Geometry check sheet. Reference: the model listing, model coordinates, mm. Face numbers are marked on the shaded views. A direction names the side the tool comes from. Give positions to 0.01 mm unless a question says otherwise; leave off trailing zeros. Write each loop counter-clockwise with the first axis right and the second up, starting at its lowest first coordinate (ties: lowest second). Pieces come first, ordered by that corner, then holes. Notation, with made-up numbers: M 69,57.25 L 127,57.25 A17 cw 127,69.25 Z; hole C -22,-1.5 d11. An arc over 180 degrees is marked long. Write each question's results on one line, items separated by ' | '.
```python
from build123d import *

# Parameters (mm, degrees)
RESSALTO_EXTRUS_O1_DEPTH = 28.35
ESBO_O3_W                = 36.7
ESBO_O3_H                = 41.8
RESSALTO_EXTRUS_O2_DEPTH = 14.75
ESBO_O5_W                = 30.5
ESBO_O5_H                = 20.5
CORTE_EXTRUS_O2_DEPTH    = 13.2
CORTE_EXTRUS_O3_DEPTH    = 69.850889609
ESBO_O7_W                = 5
ESBO_O7_H                = 16.7
CORTE_EXTRUS_O4_DEPTH    = 6.5
FILETE1_R                = 2.5
ESBO_O8_W                = 8.5
ESBO_O8_H                = 3.5
CORTE_EXTRUS_O5_DEPTH    = 14
ESBO_O9_W                = 3.2
ESBO_O9_H                = 3.2
RESSALTO_EXTRUS_O3_DEPTH = 2
ESBO_O10_R               = 10.65
RESSALTO_EXTRUS_O4_DEPTH = 17
ESBO_O11_R               = 4.25
CORTE_EXTRUS_O6_DEPTH    = 25


with BuildPart() as part:
    # Esboço1 → Ressalto-extrusão1 (new body)
    with BuildSketch(Plane.XY):
        with BuildLine():
            Line((14.1, -8.525), (14.1, 22.625))
            Line((14.1, 22.625), (-14.1, 22.625))
            Line((-14.1, 22.625), (-14.1, -8.525))
            ThreePointArc((-14.1, -8.525), (0, -22.625), (14.1, -8.525))
        make_face()
    extrude(amount=RESSALTO_EXTRUS_O1_DEPTH)

    # Esboço3 → Ressalto-extrusão2 (add)
    with BuildSketch(Plane(origin=(0, 22.625, 0), x_dir=(1, 0, 0), z_dir=(0, 1, 0))):
        with Locations((0, -7.45)):
            Rectangle(ESBO_O3_W, ESBO_O3_H)
    extrude(amount=RESSALTO_EXTRUS_O2_DEPTH)

    # Esboço5 → Corte-extrusão2 (cut)
    with BuildSketch(Plane(origin=(0, 37.375, 0), x_dir=(1, 0, 0), z_dir=(0, 1, 0))):
        with Locations((0, -13.5)):
            Rectangle(ESBO_O5_W, ESBO_O5_H)
    extrude(amount=-CORTE_EXTRUS_O2_DEPTH, mode=Mode.SUBTRACT)

    # Esboço6 → Corte-extrusão3 (cut, through all)
    with BuildSketch(Plane(origin=(0, 37.375, 0), x_dir=(1, 0, 0), z_dir=(0, 1, 0))):
        with BuildLine():
            Line((-2, 13.45), (-2, 6.30835312))
            ThreePointArc((-2, 6.30835312), (0, 4.30835312), (2, 6.30835312))
            Line((2, 6.30835312), (2, 13.45))
            Line((2, 13.45), (-2, 13.45))
        make_face()
    extrude(amount=-CORTE_EXTRUS_O3_DEPTH, mode=Mode.SUBTRACT)

    # Esboço7 → Corte-extrusão4 (cut)
    with BuildSketch(Plane(origin=(0, 37.375, 0), x_dir=(1, 0, 0), z_dir=(0, 1, 0))):
        with Locations((-9.55, 5.1)):
            Rectangle(ESBO_O7_W, ESBO_O7_H)
        with Locations((9.55, 5.1)):
            Rectangle(ESBO_O7_W, ESBO_O7_H)
    extrude(amount=-CORTE_EXTRUS_O4_DEPTH, mode=Mode.SUBTRACT)

    # Filete1
    filete1_edges = [part.edges().sort_by_distance(p)[0] for p in [
        (-12.05, 30.875, -5.1),
        (-7.05, 30.875, -5.1),
        (7.05, 30.875, -5.1),
        (12.05, 30.875, -5.1),
    ]]
    fillet(filete1_edges, radius=FILETE1_R - 0.0001)  # a hair under: the kernel refuses the full size

    # Esboço8 → Corte-extrusão5 (cut)
    with BuildSketch(Plane(origin=(0, 0, -13.45), x_dir=(-1, 0, 0), z_dir=(0, 0, -1))):
        with Locations((0.04245602, 30)):
            Rectangle(ESBO_O8_W, ESBO_O8_H)
    extrude(amount=-CORTE_EXTRUS_O5_DEPTH, mode=Mode.SUBTRACT)

    # Esboço9 → Ressalto-extrusão3 (add)
    with BuildSketch(Plane(origin=(0, 37.375, 0), x_dir=(1, 0, 0), z_dir=(0, 1, 0))):
        with Locations((-13.65, -1.65)):
            Rectangle(ESBO_O9_W, ESBO_O9_H)
        with Locations((13.65, -1.65)):
            Rectangle(ESBO_O9_W, ESBO_O9_H)
    extrude(amount=RESSALTO_EXTRUS_O3_DEPTH)

    # Esboço10 → Ressalto-extrusão4 (add)
    with BuildSketch(Plane(origin=(0, 0, 0), x_dir=(-1, 0, 0), z_dir=(0, 0, -1))):
        with Locations(Location((0, -9.125, 0), (0, 0, 180))):
            Circle(ESBO_O10_R)
    extrude(amount=RESSALTO_EXTRUS_O4_DEPTH)

    # Esboço11 → Corte-extrusão6 (cut)
    with BuildSketch(Plane(origin=(0, 0, -17), x_dir=(-1, 0, 0), z_dir=(0, 0, -1))):
        with Locations((0, -9.125)):
            Circle(ESBO_O11_R)
    extrude(amount=-CORTE_EXTRUS_O6_DEPTH, mode=Mode.SUBTRACT)


solid = part.part
```
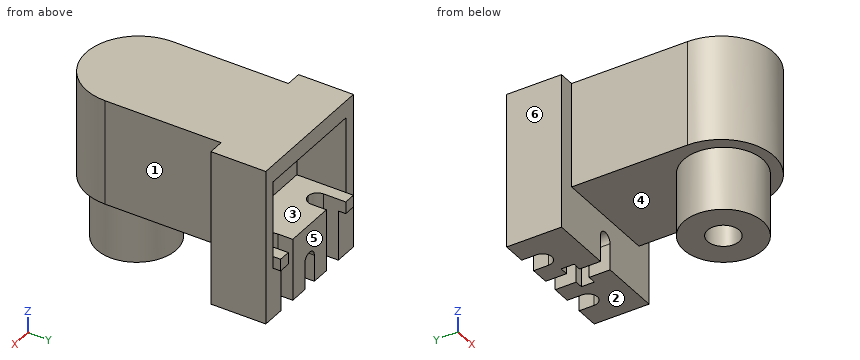
Q1. Section check B-B (x = 0). Enter the section's corners in (y, z) (3 decimals), then the cut area to 3 significant figures.
Answer key:
outline: M -22.625,0 L -19.775,0 L -19.775,-17 L -13.375,-17 L -13.375,8 L -4.875,8 L -4.875,-17 L 1.525,-17 L 1.525,0 L 22.625,0 L 22.625,-4.308 L 28.25,-4.308 L 28.25,0.55 L 31.75,0.55 L 31.75,-4.308 L 37.375,-4.308 L 37.375,3.25 L 24.175,3.25 L 24.175,23.75 L 37.375,23.75 L 37.375,28.35 L -22.625,28.35 Z | area: 1,630 mm2
Q2. Depth check by flat-ended pin: P1, Ø8, axis at y = -9, z = 17.5, coming from the +X side; P2, Ø4, axis at y = 17.5, z = 22, coming from the -X side; P3, Ø8, axis at x = 2.5, z = 15.5, coming from the +Y side (3 decimals). Enter the tip coordinate at first touch or a pass-through.
Answer key:
P1: stops at x = 14.1 | P2: stops at x = -14.1 | P3: stops at y = 24.175
Q3. Section check A-A (z = -3.5). State how many separate pieces and enclosed holes the cut face has, then the cut area to 3 significant figures.
Answer key:
separate pieces: 2 | enclosed holes: 2 | area: 752 mm2
Q4. Section check D-D (z = 22). Enter the section's corners in (x, y) (3 decimals).
Answer key:
outline: M -18.35,22.625 L -14.1,22.625 L -14.1,-8.525 A14.1 ccw 14.1,-8.525 L 14.1,22.625 L 18.35,22.625 L 18.35,37.375 L 15.25,37.375 L 15.25,24.175 L -15.25,24.175 L -15.25,37.375 L -18.35,37.375 Z
Q5. Release check for a two-part mould opening along Y. For the marked faces 4, 5 and 6 record: released by +Y, released by -Y, zero draft, split by the parting line, or undercut.
Answer key:
face 4: undercut | face 5: released by +Y | face 6: zero draft
Q6. Access from +Z, -Z, +X, -X, +Y, -Y to the whole of each face (thin tool, end or side, straight path). Record for the marked faces 1, 2 and 3.
Answer key:
face 1: +Z, -Z, +X, -Y | face 2: -Z, +X, -X, +Y | face 3: +Y
Q7. Section check C-C (z = 6). Enter the section's corners in (x, y) (3 decimals).
Answer key:
outline: M -18.35,22.625 L -14.1,22.625 L -14.1,-8.525 A14.1 ccw 14.1,-8.525 L 14.1,22.625 L 18.35,22.625 L 18.35,37.375 L 15.25,37.375 L 15.25,24.175 L -15.25,24.175 L -15.25,37.375 L -18.35,37.375 Z; hole C 0,-9.125 d8.5
Q8. Material ranges on probe 1 along Y at (x, z) = (0, -3.5) (3 decimals); probe 2 along Y at (x, z) = (0, 0.25) (3 decimals); probe 3 along Y at (x, z) = (0, -8.5) (3 decimals), recorded low to high. Write a range as [from, to].
Answer key:
probe 1: y = [-19.775, -13.375], [-4.875, 1.525], [22.625, 28.25], [31.75, 37.375] | probe 2: y = [-22.625, -13.375], [-4.875, 28.25], [31.75, 37.375] | probe 3: y = [-19.775, -13.375], [-4.875, 1.525]
